Input: part model. Units: mm. Frame: model coordinates. Face numbers are marked on the shaded views. A direction names the side the tool comes from. Round coordinates to 2 decimals unless told otherwise and drop trailing zeros. Loops run counter-clockwise (first coordinate to the right, second up) from the corner with the lowest first, then second, coordinate; pieces in that order, holes last. Notation, with made-up numbers: (78.25, -25.5) -> (98.25, -25.5) arc R30 ccw to (98.25, 3.5) -> close; hole circle Ø5 at (56, 31). An arc over 180 degrees is marked (long way). Answer in a Markdown table with one row per item. Add a question column.
Q1. Mould query, pull axis Z, two halves, no side actions, for the marked faces 1, 2 and 3. Classes: pulls with the +Z half, pulls with the -Z half, needs draft (parallel to the pull), parting line crosses it, or undercut.
Q2. Section A-A, the plane y = 7. Output: boundary loops of the cut face in (x, z), and give its area (3 significant figures).
Q3. Ray query, L1, parallel to X at y = 0.6, z = 0; L2, parallel to Y at x = -3, z = -1; L3, parallel to X at y = 3.3, z = 0. Return the intervals inside material, ascending. Write a range as from..to.
Q4. Pin query (flat end, axial travel): pin 1 (5.5 mm diameter, centred on x = 0, z = 0, fed in from -Y); pin 2 (3.5 mm diameter, centred on y = 7.5, z = 0, fed in from -X); pin 3 (5 mm diameter, centred on x = 2.5, y = 5.5, fed in from +Z); pin 4 (6 mm diameter, centred on x = 3, z = 3, fed in from +Y). Return the tip coordinate at first contact, or that it passes through.
Q5. Reachability of the marked faces 4, 5 and 6 from +Z, -Z, +X, -X, +Y, -Y: full face, straight path, thin tool, end or side. Return the list, or none.
```python
from build123d import *

# Parameters (mm, degrees)
SKETCH_1_R          = 5
SKETCH_1_R_2        = 4.5
EXTRUDE_1_DEPTH     = 1
SKETCH_1_5_R        = 4.5
SKETCH_1_5_R_2      = 4
EXTRUDE_2_DEPTH     = 2
SKETCH_1_6_R        = 4
SKETCH_1_6_W        = 5
SKETCH_1_6_H        = 5
EXTRUDE_3_DEPTH     = 10.5
CUT_EXTRUDE_START   = 10.5
SKETCH_1_7_W        = 5
SKETCH_1_7_H        = 5
CUT_EXTRUDE_1_DEPTH = 6
SKETCH_2_R          = 2.2
CUT_EXTRUDE_2_DEPTH = 20
SKETCH_3_R          = 3.75
CUT_EXTRUDE_4_DEPTH = 1
FILLET_1_R          = 1
CHAMFER_1_SIZE      = 0.3


with BuildPart() as part:
    # 스케치1 → 보스-돌출1 (new body)
    with BuildSketch(Plane(origin=(0, 0, 0), x_dir=(1, 0, 0), z_dir=(0, 1, 0))):
        with Locations(Location((0, 0, 0), (0, 0, 270))):
            Circle(SKETCH_1_R)
        with Locations(Location((0, 0, 0), (0, 0, 270))):
            Circle(SKETCH_1_R_2, mode=Mode.SUBTRACT)
    extrude(amount=EXTRUDE_1_DEPTH)

    # 스케치1<5> → 보스-돌출2 (add)
    with BuildSketch(Plane(origin=(0, 0, 0), x_dir=(1, 0, 0), z_dir=(0, 1, 0))):
        with Locations(Location((0, 0, 0), (0, 0, 270))):
            Circle(SKETCH_1_5_R)
        with Locations(Location((0, 0, 0), (0, 0, 270))):
            Circle(SKETCH_1_5_R_2, mode=Mode.SUBTRACT)
    extrude(amount=EXTRUDE_2_DEPTH)

    # 스케치1<6> → 보스-돌출3 (add)
    # profile 1 of 2: a face of its own
    with BuildSketch(Plane(origin=(0, 0, 0), x_dir=(1, 0, 0), z_dir=(0, 1, 0))):
        with Locations(Location((0, 0, 0), (0, 0, 90))):
            Circle(SKETCH_1_6_R)
        Rectangle(SKETCH_1_6_W, SKETCH_1_6_H, mode=Mode.SUBTRACT)
    # profile 2 of 2: a face of its own
    with BuildSketch(Plane(origin=(0, 0, 0), x_dir=(1, 0, 0), z_dir=(0, 1, 0))):
        Rectangle(SKETCH_1_6_W, SKETCH_1_6_H)
    extrude(amount=EXTRUDE_3_DEPTH)

    # 스케치1<7> → 컷-돌출1 (cut)
    with BuildSketch(Plane(origin=(0, 0, 0), x_dir=(1, 0, 0), z_dir=(0, 1, 0)).offset(CUT_EXTRUDE_START)):
        Rectangle(SKETCH_1_7_W, SKETCH_1_7_H)
    extrude(amount=-CUT_EXTRUDE_1_DEPTH, mode=Mode.SUBTRACT)

    # 스케치2 → 컷-돌출2 (cut)
    with BuildSketch(Plane.XZ):
        with Locations(Location((0, 0, 0), (0, 0, 270))):
            Circle(SKETCH_2_R)
    extrude(amount=-CUT_EXTRUDE_2_DEPTH, mode=Mode.SUBTRACT)

    # 스케치3 → 컷-돌출4 (cut)
    with BuildSketch(Plane.XZ):
        with Locations(Location((0, 0, 0), (0, 0, 270))):
            Circle(SKETCH_3_R)
    extrude(amount=-CUT_EXTRUDE_4_DEPTH, mode=Mode.SUBTRACT)

    # 필렛1
    fillet_1_edges = [part.edges().sort_by_distance(p)[0] for p in [
        (-2.5, 7.5, 2.5),
        (-2.5, 7.5, -2.5),
        (2.5, 7.5, -2.5),
        (2.5, 7.5, 2.5),
    ]]
    fillet(fillet_1_edges, radius=FILLET_1_R)

    # 모따기1
    chamfer_1_edges = [part.edges().sort_by_distance(p)[0] for p in [
        (0, 2, -4.5),
        (0, 1, -5),
        (0, 10.5, 4),
        (0, 0, -5),
        (0, 0, 3.75),
        (0, 1, 2.2),
        (2.5, 10.5, 0),
        (0, 10.5, 2.5),
        (-2.5, 10.5, 0),
        (0, 10.5, -2.5),
        (2.207106781, 10.5, 2.207106781),
        (-2.207106781, 10.5, 2.207106781),
        (2.207106781, 10.5, -2.207106781),
        (-2.207106781, 10.5, -2.207106781),
    ]]
    chamfer(chamfer_1_edges, length=CHAMFER_1_SIZE)


solid = part.part
```
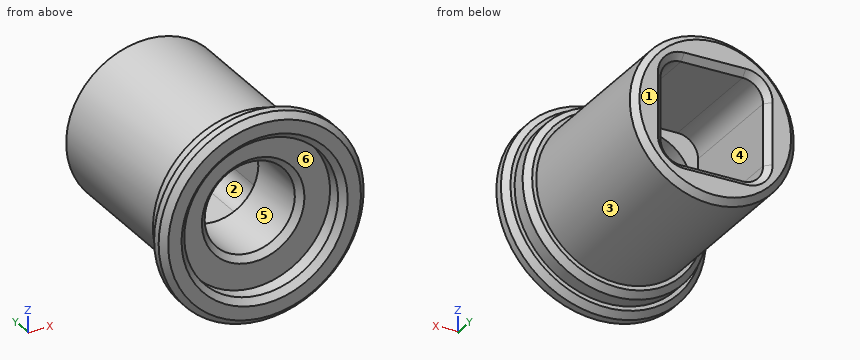
Answer block:
| question | item | result |
|---|---|---|
| 1 | face 1 | needs draft |
| 1 | face 2 | undercut |
| 1 | face 3 | parting line crosses it |
| 2 | outline | circle Ø8 at (0, 0); hole (-2.5, -1.5) arc R1 ccw to (-1.5, -2.5) -> (1.5, -2.5) arc R1 ccw to (2.5, -1.5) -> (2.5, 1.5) arc R1 ccw to (1.5, 2.5) -> (-1.5, 2.5) arc R1 ccw to (-2.5, 1.5) -> close |
| 2 | area | 26.1 mm^2 |
| 3 | L1 | -5..-3.75, 3.75..5 |
| 3 | L2 | 1..10.5 |
| 3 | L3 | -4..-2.2, 2.2..4 |
| 4 | pin 1 | y = 1 |
| 4 | pin 2 | x = -4 |
| 4 | pin 3 | z = 4 |
| 4 | pin 4 | y = 10.5 |
| 5 | face 4 | +Y |
| 5 | face 5 | +Y, -Y |
| 5 | face 6 | -Y |
